from build123d import *

# Parameters (mm, degrees)
SKETCH_7_R          = 0.325
EXTRUDE_1_DEPTH     = 5
SKETCH_8_R          = 2.5
CUT_EXTRUDE_1_DEPTH = 0.2


with BuildPart() as part:
    # Эскиз6 → Повернуть1 (revolve)
    with BuildSketch(Plane.XY):
        Polygon((0, 13), (0, 0), (3.1, 0), (4.6, 1.5), (4.6, 3.812414318), (3.912414318, 4.5), (3.912414318, 8.5), (4.6, 9.187585682), (4.6, 11.5), (3.1, 13), align=None)
    revolve(axis=Axis((0, 13, 0), (0, -1, 0)))

    # Эскиз7 → Бобышка-Вытянуть1 (add)
    with BuildSketch(Plane.XZ):
        with Locations((2.5, 0)):
            Circle(SKETCH_7_R)
        with Locations((-2.5, 0)):
            Circle(SKETCH_7_R)
    extrude(amount=EXTRUDE_1_DEPTH)

    # Эскиз8 → Вырез-Вытянуть1 (cut)
    with BuildSketch(Plane(origin=(0, 13, 0), x_dir=(1, 0, 0), z_dir=(0, 1, 0))):
        Circle(SKETCH_8_R)
    extrude(amount=-CUT_EXTRUDE_1_DEPTH, mode=Mode.SUBTRACT)


solid = part.part
The model under review builds one solid part; all positions refer to its coordinate system, in mm. A direction names the side the tool comes from. Give positions to 0.01 mm unless a question says otherwise; leave off trailing zeros. Loops run counter-clockwise (first coordinate to the right, second up) from the corner with the lowest first, then second, coordinate; pieces in that order, holes last. Notation, with made-up numbers: (78.25, 56) -> (87.25, 56) arc R13 ccw to (87.25, 62) -> close; hole circle Ø8 at (14, -16.75). An arc over 180 degrees is marked (long way). Answer as a JSON object with one key per item and string values. Group by question number.
Q1. Insertion check: pin 1 (1.5 mm diameter, centred on y = 5.5, z = -1.5, fed in from +X); pin 2 (1.5 mm diameter, centred on x = 1, z = 0, fed in from +Y); pin 3 (5 mm diameter, centred on y = -2.5, z = -2, fed in from -X) (3 decimals). Each pin has a flat end and moves straight along its axis. Give the tip position at first contact, or say it passes through.
Q2. Take a section at A-A (z = 0). Write out the cut boundary in (x, y) (3 decimals), plus the area to 3 significant figures.
Q3. Wall thickness on line 1 along Z through (x, y) = (0, 12.9); line 2 along Z through (x, y) = (0, 12.95): over which ranges is each line inside the solid? List them lowest first.
Q4. Take a section at B-B (y = -3.25). Write out the cut boundary in (x, z) (3 decimals).
Q5. Tool access review of faces 1 (the cylindrical face through (-3.65, 2.67, -2.8)), 2 (the cylindrical face through (1.81, 6.53, -3.47)): name each direction out of +Z, -Z, +X, -X, +Y, -Y from which nothing blocks a thin tool from reaching the whole face with its end or side.
Q6. Draft analysis for pull direction X (two halves, no side actions). For faces 3 (the cylindrical face through (-3.65, 10.36, -2.8)), 4 (the flat face through (0, 12.8, 0)), state which applies: pulls with the +X half, pulls with the -X half, needs draft (parallel to the pull), parting line crosses it, or undercut.
Q7. Take a section at D-D (y = 2.75). Write out the cut boundary in (x, z).
Q8. Take a section at C-C (x = 0). Write out the cut boundary in (y, z), plus the area to 3 significant figures.
Answer below:
{
 "1": {"pin 1": "stops at x = 3.84", "pin 2": "stops at y = 12.8", "pin 3": "stops at x = -2.825"},
 "2": {"outline": "(-4.6, 1.5) -> (-3.1, 0) -> (-2.825, 0) -> (-2.825, -5) -> (-2.175, -5) -> (-2.175, 0) -> (2.175, 0) -> (2.175, -5) -> (2.825, -5) -> (2.825, 0) -> (3.1, 0) -> (4.6, 1.5) -> (4.6, 3.812) -> (3.912, 4.5) -> (3.912, 8.5) -> (4.6, 9.188) -> (4.6, 11.5) -> (3.1, 13) -> (2.5, 13) -> (2.5, 12.8) -> (-2.5, 12.8) -> (-2.5, 13) -> (-3.1, 13) -> (-4.6, 11.5) -> (-4.6, 9.188) -> (-3.912, 8.5) -> (-3.912, 4.5) -> (-4.6, 3.812) -> close", "area": "114 mm2"},
 "3": {"line 1": "z = -3.2 to -2.5, 2.5 to 3.2", "line 2": "z = -3.15 to -2.5, 2.5 to 3.15"},
 "4": {"outline": "circle Ø0.65 at (-2.5, 0); circle Ø0.65 at (2.5, 0)"},
 "5": {"face 1": "+Y, -Y", "face 2": "none"},
 "6": {"face 3": "parting line crosses it", "face 4": "undercut"},
 "7": {"outline": "circle Ø9.2 at (0, 0)"},
 "8": {"outline": "(0, -3.1) -> (1.5, -4.6) -> (3.81, -4.6) -> (4.5, -3.91) -> (8.5, -3.91) -> (9.19, -4.6) -> (11.5, -4.6) -> (13, -3.1) -> (13, -2.5) -> (12.8, -2.5) -> (12.8, 2.5) -> (13, 2.5) -> (13, 3.1) -> (11.5, 4.6) -> (9.19, 4.6) -> (8.5, 3.91) -> (4.5, 3.91) -> (3.81, 4.6) -> (1.5, 4.6) -> (0, 3.1) -> close", "area": "108 mm2"}
}
